Autodesk Inventor part; units mm, degrees
ref_plane "YZ Plane" through (0, 0, 0) normal (1, 0, 0) x (0, 1, 0)
ref_plane "XZ Plane" through (0, 0, 0) normal (0, 1, 0) x (-1, 0, 0)
ref_plane "XY Plane" through (0, 0, 0) normal (0, 0, 1) x (1, 0, 0)
ref_plane "Work Plane1" through (-106.5416, 98.4713, 124.9427) normal (0, 0, 1) x (1, 0, 0)
sketch "Sketch1" plane through (-106.5416, 98.4713, 124.9427) normal (0, 0, 1) x (1, 0, 0)
  circle A0 centre (19.5, 13) radius 1.5
  arc A1 (52.5, 10.25) -> (37.5, 10.25) centre (45, 10.25) ccw
  circle A2 centre (19.5, 13) radius 5.5 construction
  line L0 (45, 10.25) -> (45, 17.75) construction
  line L1 (45, 17.75) -> (45, 23.75) construction
  line L2 (45, 23.75) -> (19.5, 23.75) construction
  arc A3 (14.0371, 13.6378) -> (25, 13) centre (19.5, 13) ccw
  line L3 (25, 13) -> (25, 23.75)
  circle A4 centre (19.5, 13) radius 1.5
  line L4 (14.0028, 12.8238) -> (14.0028, 23.75)
  line L5 (14.0028, 23.75) -> (25, 23.75)
  point P0 (106.5416, -98.4713)
  point P1 (14.0469, 12.2829)
  dimension "d0" = 11
  dimension "d4" = 10.75
extrude "Extrusion1" add sketch "Sketch1" along normal blind 8
pattern_linear "Rectangular Pattern2" count 2 spacing 51 along (1, 0, 0) count 2 spacing 20 along (0, 0, -1) of "Extrusion1"
sketch "Sketch3" plane through (-92.5388, 122.2213, 124.9427) normal (0, 1, 0) x (1, 0, 0)
  line L0 (0, 20) -> (61.9972, 20) construction
  line L1 (0, 20) -> (0, -8) construction
  line L2 (0, 6) -> (86.2224, 6) construction
  line L3 (31, 37) -> (31, -25) construction
  line L4 (31, -25) -> (-14.75, -25) construction
  line L5 (31, -25) -> (76.75, -25) construction
  line L6 (76.75, -25) -> (76.75, 37)
  line L7 (76.75, 37) -> (-14.75, 37)
  line L8 (-14.75, 37) -> (-14.75, -25)
  line L9 (-14.75, -25) -> (76.75, -25)
  point P0 (92.5388, 124.9427)
  dimension "d29" = 45.75
  dimension "d30" = 45.75
  dimension "d31" = 62
extrude "Extrusion3" add sketch "Sketch3" against normal blind 5
ref_plane "Work Plane2" through (-60.8166, 113.6367, 119.7132) normal (0, 0.9135, -0.4067) x (-1, 0, 0)
sketch "Sketch4" plane through (-60.8166, 113.6367, 119.7132) normal (0, 0.9135, -0.4067) x (-1, 0, 0)
  circle A0 centre (-0.457, 0.457) radius 0.457
  circle A1 centre (-0.457, 0.457) radius 0.457
  circle A2 centre (-0.457, 0.457) radius 0.375
  point P0 (-60.8166, -155.5837)
  dimension "d32" = 0.75
extrude "Extrusion4" cut sketch "Sketch4" along normal blind 15 contours A2
pattern_linear "Rectangular Pattern3" count 2 spacing 4 along (0, 0, -1) of "Extrusion4"
sketch "Sketch5" plane through (-107.2888, 122.2213, 149.9427) normal (0, 1, 0) x (1, 0, 0)
  line L0 (0, 0) -> (0, 62)
  line L1 (0, 62) -> (91.5, 62)
  line L2 (0, 62) -> (0, 51)
  line L3 (0, 51) -> (8, 51)
  line L4 (8, 51) -> (8, 62)
  line L5 (0, 62) -> (8, 62)
  point P0 (107.2888, 149.9427)
  dimension "d38" = 11
  dimension "d39" = 8
extrude "Extrusion5" add sketch "Sketch5" along normal blind 13.5
sketch "Sketch6" plane through (-99.2888, 122.2213, 98.9427) normal (1, 0, 0) x (0, 0, -1)
  line L0 (11, 0) -> (11, 13.5)
  line L1 (0, 13.5) -> (11, 13.5)
  circle A0 centre (5.5, 8) radius 1.5
  dimension "d42" = 3
  dimension "d43" = 5.5
  dimension "d44" = 5.5
extrude "Extrusion6" cut sketch "Sketch6" against normal blind 24.6
fillet "Fillet1" radius 3 2 edges at (-103.2888, 135.7213, 98.9427) (-103.2888, 135.7213, 87.9427)
pattern_linear "Rectangular Pattern4" count 2 spacing 51 along (0, 0, 1) count 2 spacing 83.5 along (1, 0, 0) of "Extrusion5", "Fillet1", "Extrusion6"
Read the model definition and answer for the solid it produces. Units are mm, in the model's axes. A direction names the side the tool comes from. Coordinates: 2 decimals unless noted, no trailing zeros. Write each loop counter-clockwise with the first axis right and the second up, starting at its lowest first coordinate (ties: lowest second). Pieces come first, ordered by that corner, then holes. Notation, with made-up numbers: (84.5, 23.25) -> (101.5, 23.25) arc R19 cw to (101.5, 47.25) -> close; hole circle Ø10 at (50, 77). An arc over 180 degrees is marked (long way). Write item = value, one per line.
(1) Given pin 1 Ø6 at (x, z) = (-41, 117.5) entering from -Y; pin 2 Ø4 at (x, y) = (-78.5, 126) entering from +Z; pin 3 Ø5.5 at (x, y) = (-85, 111) entering from +Z; pin 4 Ø18.5 at (x, z) = (-56.5, 119.5) entering from +Y, each flat-ended and moving along its own axis, determine where each tip first touches the part or whether it passes through.
From the geometry:
pin_1 = 117.22
pin_2 = through
pin_3 = 132.94
pin_4 = 122.22
(2) Section C-C on x = -22.5 is taken. Write down the section's boundary in (y, z), plus the area to 3 significant figures.
From the geometry:
outline = (117.22, 87.94) -> (132.72, 87.94) arc R3 ccw to (135.72, 90.94) -> (135.72, 95.94) arc R3 ccw to (132.72, 98.94) -> (122.22, 98.94) -> (122.22, 138.94) -> (132.72, 138.94) arc R3 ccw to (135.72, 141.94) -> (135.72, 146.94) arc R3 ccw to (132.72, 149.94) -> (117.22, 149.94) -> close; hole circle Ø3 at (130.22, 93.44); hole circle Ø3 at (130.22, 144.44)
area = 585 mm2
(3) Section A-A on y = 124.5 is taken. Write down the section's boundary in (x, z), plus the area to 3 significant figures.
From the geometry:
outline = (-107.29, 87.94) -> (-99.29, 87.94) -> (-99.29, 98.94) -> (-107.29, 98.94) -> close; (-107.29, 138.94) -> (-99.29, 138.94) -> (-99.29, 149.94) -> (-107.29, 149.94) -> close; (-23.79, 87.94) -> (-15.79, 87.94) -> (-15.79, 98.94) -> (-23.79, 98.94) -> close; (-23.79, 138.94) -> (-15.79, 138.94) -> (-15.79, 149.94) -> (-23.79, 149.94) -> close
area = 352 mm2
(4) Which of the six approach directions +Z, -Z, +X, -X, +Y, -Y give full straight-line access (tool end or side, diameter ignored) to faces 1 (the face through (-92.539, 114, 129)), 2 (the face through (-37, 113, 104.943)), 3 (the face through (-41.539, 114, 109)), 4 (the face through (-88, 113, 132.943))?
From the geometry:
face_1 = +Z, -Z, -X, -Y
face_2 = -Z, +X, -X, -Y
face_3 = +Z, -Z, -Y
face_4 = +Z, +X, -X, -Y
(5) Section D-D on z = 131.5 is taken. Write down the section's boundary in (x, y), plus the area to 3 significant figures.
From the geometry:
outline = (-107.29, 117.22) -> (-92.54, 117.22) -> (-92.54, 111.3) arc R5.5 ccw to (-81.54, 111.47) -> (-81.54, 117.22) -> (-41.54, 117.22) -> (-41.54, 111.3) arc R5.5 ccw to (-30.54, 111.47) -> (-30.54, 117.22) -> (-15.79, 117.22) -> (-15.79, 122.22) -> (-107.29, 122.22) -> close; hole circle Ø3 at (-87.04, 111.47); hole circle Ø3 at (-36.04, 111.47)
area = 665 mm2
(6) Straight lines are drawn through the part: L1, parallel to Z at x = -35, y = 113.25; L2, parallel to X at y = 123.5, z = 145; L3, parallel to Y at x = -42.5, z = 99. For each, find the intervals that lie inside material, in ascending order. Write a range as from..to.
From the geometry:
L1 = 104.94..112.94, 124.94..132.94
L2 = -107.29..-99.29, -23.79..-15.79
L3 = 117.22..122.22
(7) Section B-B on z = 144 is taken. Write down the section's boundary in (x, y).
From the geometry:
outline = (-107.29, 117.22) -> (-15.79, 117.22) -> (-15.79, 128.79) -> (-23.79, 128.79) -> (-23.79, 122.22) -> (-99.29, 122.22) -> (-99.29, 128.79) -> (-107.29, 128.79) -> close; (-107.29, 131.65) -> (-99.29, 131.65) -> (-99.29, 135.72) -> (-107.29, 135.72) -> close; (-23.79, 131.65) -> (-15.79, 131.65) -> (-15.79, 135.72) -> (-23.79, 135.72) -> close
(8) For a pull along Z with two mould halves and no side action, classify faces 5 (the face through (-103.23, 134.82, 139.8)), 6 (the face through (-103, 127, 98.943)), 7 (the face through (-19.733, 134.866, 149.041)), 8 (the face through (-15.789, 120, 119)) as +Z half, -Z half, draft (parallel to the pull), parting line (faces both ways), or undercut.
From the geometry:
face_5 = undercut
face_6 = undercut
face_7 = +Z half
face_8 = draft
